Design review of the part shown in the three views and the two pictorial views. Dimensions are in mm from the part's minimum x, y and z. A direction names the side the tool comes from. Give positions to 0.01 mm unless a question says otherwise; leave off trailing zeros. Loops run counter-clockwise (first coordinate to the right, second up) from the corner with the lowest first, then second, coordinate; pieces in that order, holes last. Notation, with made-up numbers: (73.25, 10.25) -> (83.25, 10.25) arc R23 cw to (83.25, 44.25) -> close; hole circle Ø6 at (58, -7.75). An arc over 180 degrees is marked (long way). One line per question, with ' | ' between items. Start each with the question number.
(1) Consider section D-D (z = 12.5). Write out the cut boundary in (x, y) (1 decimal), and give its area (3 significant figures).
(2) Draft analysis for pull direction Z (two halves, no side actions). For the marked faces 4, 5, 6 and 7, state which applies: +Z half, -Z half, draft (parallel to the pull), parting line (faces both ways), or undercut.
(3) Consider section B-B (z = 40). Write out the cut boundary in (x, y) (1 decimal), and give its area (3 significant figures).
(4) Tool access review of the marked faces 1, 2 and 3: name each direction out of +Z, -Z, +X, -X, +Y, -Y from which nothing blocks a thin tool from reaching the whole face with its end or side.
(5) Consider section A-A (x = 32.5). Write out the cut boundary in (y, z).
(6) Insertion check: P1, Ø3, axis at y = 6, z = 25, coming from the +X side. The pin has a flat end and moves straight along its axis. Give the tip position at first contact, or say it passes through.
(7) Consider section C-C (y = 6.5). Write out the cut boundary in (x, z) (1 decimal), and give its area (3 significant figures).
(8) Wall thickness on probe 1 along X at (y, z) = (2, 8) (1 decimal); probe 2 along Z at (x, y) = (47, 0.5); probe 3 along X at (y, z) = (1, 13) (1 decimal): over which ranges is each line inside the solid? List them lowest first.
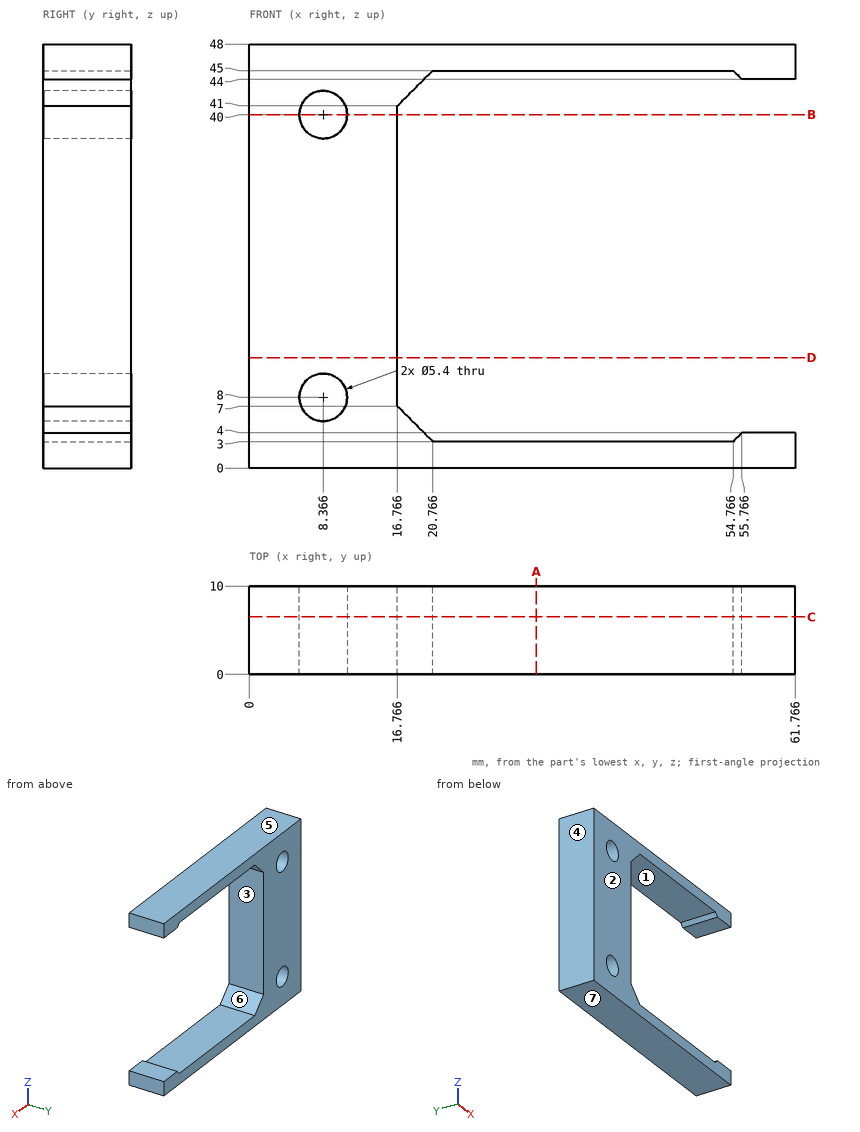
A:
1) outline: (0, 0) -> (16.8, 0) -> (16.8, 10) -> (0, 10) -> close | area: 168 mm^2
2) face 4: draft | face 5: +Z half | face 6: undercut | face 7: -Z half
3) outline: (0, 0) -> (5.7, 0) -> (5.7, 10) -> (0, 10) -> close; (11.1, 0) -> (16.8, 0) -> (16.8, 10) -> (11.1, 10) -> close | area: 114 mm^2
4) face 1: +Y, -Y | face 2: +Z, -Z, +X, -X, -Y | face 3: +X, +Y, -Y
5) outline: (0, 0) -> (10, 0) -> (10, 3) -> (0, 3) -> close; (0, 45) -> (10, 45) -> (10, 48) -> (0, 48) -> close
6) P1: stops at x = 16.77
7) outline: (0, 0) -> (61.8, 0) -> (61.8, 4) -> (55.8, 4) -> (54.8, 3) -> (20.8, 3) -> (16.8, 7) -> (16.8, 41) -> (20.8, 45) -> (54.8, 45) -> (55.8, 44) -> (61.8, 44) -> (61.8, 48) -> (0, 48) -> close; hole circle Ø5.4 at (8.4, 8); hole circle Ø5.4 at (8.4, 40) | area: 1,060 mm^2
8) probe 1: x = 0 to 5.7, 11.1 to 16.8 | probe 2: z = 0 to 3, 45 to 48 | probe 3: x = 0 to 16.8
